The listing builds one solid part. Answer for the finished solid, in the listing's coordinates (mm). Coordinates: 2 decimals unless noted, no trailing zeros. Order: outer loops, then holes, each group sorted by start corner. A loop starts at its lowest first (then second) coordinate and runs counter-clockwise, first axis right, second up. Notation, with made-up numbers: (69.25, 32) -> (128.25, 32) arc R16 ccw to (128.25, 60) -> close; hole circle Ø2 at (-5, -25.75). An arc over 180 degrees is marked (long way). One line per question, with ' | ' between items.
Autodesk Inventor part; units mm, degrees
ref_plane "YZ Plane" through (0, 0, 0) normal (1, 0, 0) x (0, 1, 0)
ref_plane "XZ Plane" through (0, 0, 0) normal (0, 1, 0) x (-1, 0, 0)
ref_plane "XY Plane" through (0, 0, 0) normal (0, 0, 1) x (1, 0, 0)
sketch "Sketch1" plane through (0, 0, 0) normal (0, 1, 0) x (-1, 0, 0)
  circle A0 centre (0, 0) radius 11.125
  circle A1 centre (0, 0) radius 15
  dimension "d0" = 22.25
  dimension "d1" = 30
extrude "Extrusion1" add sketch "Sketch1" along normal blind 7
sketch "Sketch2" plane through (0, 7, 0) normal (0, 1, 0) x (1, 0, 0)
  circle A0 centre (0, 0) radius 13.625
  circle A1 centre (0, 0) radius 15
  dimension "d4" = 30
extrude "Extrusion2" add sketch "Sketch2" against normal blind 3
sketch "Sketch3" plane through (0, 0, 0) normal (0, -1, 0) x (1, 0, 0)
  circle A0 centre (0, 0) radius 13.625
  circle A1 centre (0, 0) radius 15
  dimension "d7" = 30
extrude "Extrusion3" add sketch "Sketch3" against normal blind 3
sketch "Sketch4" plane through (0, 7, 0) normal (0, 1, 0) x (1, 0, 0)
  circle A0 centre (0, 0) radius 15
  circle A1 centre (0, 0) radius 16.5
  dimension "d12" = 33
extrude "Extrusion4" add sketch "Sketch4" against normal blind 3
sketch "Sketch5" plane through (0, 0, 0) normal (0, -1, 0) x (1, 0, 0)
  circle A0 centre (0, 0) radius 15
  circle A1 centre (0, 0) radius 16.5
extrude "Extrusion5" add sketch "Sketch5" against normal blind 3
fillet "Fillet3" radius 2 1 edges at (-16.5, 4, 0)
fillet "Fillet4" radius 2 1 edges at (-16.5, 3, 0)
properties part number "OutterBearing"
Item 1: Section B-B, the plane x = 0 is taken. Give the vertices of the cut face in (y, z) (1 decimal), plus the area to 3 significant figures.
Computed values:
outline: (0, -16.5) -> (1.1, -16.5) arc R2 ccw to (3, -15) -> (4, -15) arc R2 ccw to (5.9, -16.5) -> (7, -16.5) -> (7, -11.1) -> (0, -11.1) -> close; (0, 11.1) -> (7, 11.1) -> (7, 16.5) -> (5.9, 16.5) arc R2 ccw to (4, 15) -> (3, 15) arc R2 ccw to (1.1, 16.5) -> (0, 16.5) -> close | area: 69.2 mm^2
Item 2: Section D-D, the plane y = 5.5 is taken. Give the vertices of the cut face in (x, z) (3 decimals).
Computed values:
outline: circle Ø32.904 at (0, 0); hole circle Ø22.25 at (0, 0)
Item 3: Each of these flat-tipped pins is pushed along its axis until it touches: pin 1 Ø1.5 at (x, z) = (-5.5, 7) entering from -Y; pin 2 Ø10 at (x, z) = (7, 9) entering from -Y; pin 3 Ø2 at (x, y) = (-11, 5) entering from +Z; pin 4 Ø1 at (y, z) = (1, 8) entering from +X. Where does it stop, or does it pass through?
Computed values:
pin 1: passes through | pin 2: stops at y = 0 | pin 3: stops at z = 12.97 | pin 4: stops at x = 14.7
Item 4: Section C-C, the plane y = 0.5 is taken. Give the vertices of the cut face in (x, z) (3 decimals).
Computed values:
outline: circle Ø33 at (0, 0); hole circle Ø22.25 at (0, 0)
Item 5: Find the intervals of material crossed by L1, parallel to Z at x = 0, y = 3.25 (3 decimals); L2, parallel to X at y = 3.25, z = 8; L3, parallel to Z at x = -4, y = 4.25, in increasing order.
Computed values:
L1: z = -15 to -11.125, 11.125 to 15 | L2: x = -12.69 to -7.73, 7.73 to 12.69 | L3: z = -15.05 to -10.38, 10.38 to 15.05
Item 6: Section A-A, the plane z = 0 is taken. Give the vertices of the cut face in (x, y) (1 decimal).
Computed values:
outline: (-16.5, 0) -> (-11.1, 0) -> (-11.1, 7) -> (-16.5, 7) -> (-16.5, 5.9) arc R2 ccw to (-15, 4) -> (-15, 3) arc R2 ccw to (-16.5, 1.1) -> close; (11.1, 0) -> (16.5, 0) -> (16.5, 1.1) arc R2 ccw to (15, 3) -> (15, 4) arc R2 ccw to (16.5, 5.9) -> (16.5, 7) -> (11.1, 7) -> close
Item 7: Determine the mould class of faces 1 (the face through (14.985, 3.493, -0.66)), 2 (the face through (15.24, 0.52, -6.32)), 3 (the face through (11, 7, 3)), 4 (the face through (11, 0, -3)) for opening direction Y: pulls with the +Y half, pulls with the -Y half, needs draft (parallel to the pull), parting line crosses it, or undercut.
Computed values:
face 1: undercut | face 2: needs draft | face 3: pulls with the +Y half | face 4: pulls with the -Y half
